Input: part model. Units: mm. Frame: model coordinates. Round coordinates to 2 decimals unless told otherwise and drop trailing zeros. Order: outer loops, then holes, each group sorted by start corner. A loop starts at its lowest first (then second) coordinate and runs counter-clockwise, first axis right, second up. Notation, with made-up numbers: M 38.5,37 L 61.5,37 A28 cw 61.5,67 Z; hole C -24.75,70 d1. An arc over 180 degrees is marked long. One line per question, with ' | ' between items.
```python
from build123d import *

# Parameters (mm, degrees)
PAD_DEPTH = 10
FILLET_R  = 2


with BuildPart() as part:
    # Sketch → Pad (new body)
    with BuildSketch(Plane.XY):
        Polygon((-30, 54.378467), (30, 54.378467), (55.357096, 0), (30, -54.378467), (-30, -54.378467), (-55.357096, 0), align=None)
    extrude(amount=PAD_DEPTH)

    # Fillet
    fillet_edges = [part.edges().sort_by_distance(p)[0] for p in [
        (30, 54.378467, 5),
        (-30, 54.378467, 5),
        (-55.357096, 0, 5),
        (-30, -54.378467, 5),
        (30, -54.378467, 5),
        (55.357096, 0, 5),
    ]]
    fillet(fillet_edges, radius=FILLET_R)


solid = part.part
```
Item 1: Line query: line 1 along X through (y, z) = (-41.5, 3); line 2 along Y through (x, z) = (47.5, 0.5); line 3 along X through (y, z) = (2.5, 6). Output: solid intervals per line, ascending. Write a range as from..to.
Report:
line 1: -36.01..36.01 | line 2: -16.85..16.85 | line 3: -54.19..54.19
Item 2: Section query B-B, the plane y = -38. Return loops of the section in (x, z).
Report:
outline: M -37.64,0 L 37.64,0 L 37.64,10 L -37.64,10 Z
Item 3: Section query A-A, the plane z = 5.75. Return loops of the section in (x, y), plus the area to 3 significant figures.
Report:
outline: M -54.96,-0.85 L -30.54,-53.22 A2 ccw -28.73,-54.38 L 28.73,-54.38 A2 ccw 30.54,-53.22 L 54.96,-0.85 A2 ccw 54.96,0.85 L 30.54,53.22 A2 ccw 28.73,54.38 L -28.73,54.38 A2 ccw -30.54,53.22 L -54.96,0.85 A2 ccw Z | area: 9,280 mm²
Item 4: First-contact query: pin 1 (1.5 mm diameter, centred on x = 33.5, z = 4, fed in from +Y); pin 2 (1 mm diameter, centred on x = -42, z = 8, fed in from +Y); pin 3 (1.5 mm diameter, centred on y = -40.5, z = 2, fed in from +X). Flat tips, straight axial feed; report the tip coordinate or a pass-through.
Report:
pin 1: y = 48.48 | pin 2: y = 29.72 | pin 3: x = 36.82
Item 5: Section query C-C, the plane x = -41. Return loops of the section in (y, z).
Report:
outline: M -30.79,0 L 30.79,0 L 30.79,10 L -30.79,10 Z
